For this review, take the finished solid that the model builds, in its own axes (mm). A direction names the side the tool comes from. Give positions to 0.01 mm unless a question says otherwise; leave off trailing zeros. Loops run counter-clockwise (first coordinate to the right, second up) from the corner with the lowest first, then second, coordinate; pieces in that order, holes last.
```python
from build123d import *

# Parameters (mm, degrees)
BOSS_EXTRUDE2_OUTLINE_R = 1.6
BOSS_EXTRUDE2_DEPTH     = 7
CUT_EXTRUDE1_DEPTH      = 58.280013967


# Read off the part's stored shape, not the designer's step: Boss-Extrude2
with BuildPart() as part:
    # Boss-Extrude2 outline → Boss-Extrude2 (new body)
    with BuildSketch(Plane(origin=(0, 0, 0), x_dir=(1, 0, 0), z_dir=(0, 1, 0))):
        with BuildLine():
            ThreePointArc((36, 20), (43.304735803, 31.262029255), (30.042934529, 33.339791286))
            ThreePointArc((30.042934529, 33.339791286), (3.05899236, 29.845703842), (-23.704753961, 34.749137831))
            ThreePointArc((-23.704753961, 34.749137831), (-35.680921255, 30.236838992), (-28, 20))
            ThreePointArc((-28, 20), (-15.417509156, 12.586209164), (-7.999997816, 0.005911236))
            ThreePointArc((-7.999997816, 0.005911236), (-0.002955618, -7.999999454), (8, 0))
            ThreePointArc((8, 0), (19.451858394, 13.567398249), (36, 20))
        make_face()
        Circle(BOSS_EXTRUDE2_OUTLINE_R, mode=Mode.SUBTRACT)
        with Locations((-28, 28)):
            Circle(BOSS_EXTRUDE2_OUTLINE_R, mode=Mode.SUBTRACT)
        with Locations((36, 28)):
            Circle(BOSS_EXTRUDE2_OUTLINE_R, mode=Mode.SUBTRACT)
    extrude(amount=BOSS_EXTRUDE2_DEPTH)

    # Sketch5 → Cut-Extrude1 (cut, through all)
    with BuildSketch(Plane(origin=(0, 7, 0), x_dir=(1, 0, 0), z_dir=(0, 1, 0))):
        Polygon((-11.978854601, 22.378102142), (-11.893313223, 24.821105741), (-13.966245712, 26.116688546), (-16.124719579, 24.969267753), (-16.210260957, 22.526264155), (-14.137328468, 21.230681349), align=None)
        Polygon((19.546993666, 22.594588654), (18.156731561, 25.002593256), (15.37620735, 25.002593256), (13.985945245, 22.594588654), (15.37620735, 20.186584052), (18.156731561, 20.186584052), align=None)
        Polygon((0, 8.213063469), (3.066820834, 9.983693303), (3.066820834, 13.524952971), (0, 15.295582806), (-3.066820834, 13.524952971), (-3.066820834, 9.983693303), align=None)
    extrude(amount=-CUT_EXTRUDE1_DEPTH, mode=Mode.SUBTRACT)


solid = part.part
```
Q1. For pin 1 Ø3 at (y, z) = (2.5, -12.5) entering from -X; pin 2 Ø3 at (x, y) = (-26.5, 3.5) entering from +Z; pin 3 Ø1.5 at (y, z) = (4, -23) entering from +X, all flat-tipped, find the tip position at first contact; note any pin that passes through.
Answers:
pin 1: stops at x = -16.94
pin 2: stops at z = -18.96
pin 3: stops at x = 42.78
Q2. Machinability: for faces 5 (the cylindrical face through (3.441, 3.451, -29.837)), 6 (the flat face through (1.512, 3.549, -9.086)), which of the approach directions +Z, -Z, +X, -X, +Y, -Y give a long, thin tool a straight path to every point of the face, cutting with its end or side? Answer none if there is none.
Answers:
face 5: -Z, +Y, -Y
face 6: +Y, -Y
Q3. Consider section C-C on x = -4.5. Give the boundary of the cut face in (y, z), plus the area to 3 significant figures.
Answers:
outline: (0, -30.37) - (7, -30.37) - (7, 6.61) - (0, 6.61) - close
area: 259 mm2
Q4. Consider section A-A on z = -31. Give the boundary of the cut face in (x, y), plus the area to 3 significant figures.
Answers:
outline: (-35.42, 0) - (-9.03, 0) - (-9.03, 7) - (-35.42, 7) - close; (19.77, 0) - (43.42, 0) - (43.42, 7) - (19.77, 7) - close
area: 350 mm2
Q5. Consider section D-D on z = -3. Give the boundary of the cut face in (x, y).
Answers:
outline: (-9.04, 0) - (9.64, 0) - (9.64, 7) - (-9.04, 7) - close
Q6. For probe 1 along X at (y, z) = (2.5, -28); probe 2 along Z at (x, y) = (0, 3.75); probe 3 along X at (y, z) = (5, -22), list the stretches that pass through material, from the lowest coordinate up.
Answers:
probe 1: x = -36 to -29.6, -26.4 to 34.4, 37.6 to 44
probe 2: z = -29.98 to -15.3, -8.21 to -1.6, 1.6 to 8
probe 3: x = -33.29 to -15.37, -12.69 to 14.33, 19.2 to 41.29
Q7. Mouldability with a two-part tool opening along X and no side actions: class faces 1 (the cylindrical face through (-15.56, 3.45, -12.73)), 2 (the flat face through (1.55, 3.55, -14.4)), 3 (the flat face through (3, 7, -19)), 4 (the cylindrical face through (0, 3, 8)) as +X half, -X half, draft (parallel to the pull), parting line (faces both ways), or undercut.
Answers:
face 1: -X half
face 2: undercut
face 3: draft
face 4: parting line
Q8. Consider section B-B on y = 3. Give the boundary of the cut face in (x, z), plus the area to 3 significant figures.
Answers:
outline: (-28, -20) arc R8 ccw (long way) to (-23.7, -34.75) arc R88.13 cw to (30.04, -33.34) arc R8 ccw (long way) to (36, -20) arc R35.95 cw to (8, 0) arc R8 ccw to (-8, -0.01) arc R29.2 cw to start; hole circle Ø3.2 at (-28, -28); hole (-16.21, -22.53) - (-16.12, -24.97) - (-13.97, -26.12) - (-11.89, -24.82) - (-11.98, -22.38) - (-14.14, -21.23) - close; hole (-3.07, -13.52) - (0, -15.3) - (3.07, -13.52) - (3.07, -9.98) - (0, -8.21) - (-3.07, -9.98) - close; hole circle Ø3.2 at (0, 0); hole (13.99, -22.59) - (15.38, -25) - (18.16, -25) - (19.55, -22.59) - (18.16, -20.19) - (15.38, -20.19) - close; hole circle Ø3.2 at (36, -28)
area: 1,600 mm2
